```python
from build123d import *

# Parameters (mm, degrees)
SKIZZE1_R                       = 1.6
AUFSATZ_LINEAR_AUSTRAGEN1_DEPTH = 10


with BuildPart() as part:
    # Skizze1 → Aufsatz-Linear austragen1 (new body)
    with BuildSketch(Plane.XY):
        Polygon((5, 9.999223218), (4.999950827, 19.975708513), (-1, 19.999999998), (-1, 29.999223216), (5, 29.999223216), (4.999950827, 39.975708511), (-1, 39.999999996), (-1, 49.999223214), (5, 49.999223214), (4.999950827, 59.975708509), (-1, 59.999999994), (-1, 69.999223211), (5, 70), (4.999950827, 79.975708506), (-1, 79.999999991), (-1, 89.999223209), (5, 90), (4.999950827, 99.975708504), (-1, 99.999999989), (-1, 109.999223207), (5, 110), (4.999950827, 119.975708502), (-1, 119.999999987), (-1, 129.999223205), (5, 130), (4.999950827, 139.9757085), (-1, 139.999999985), (-1, 149.999223203), (5, 150), (4.999950827, 159.975708498), (-1, 159.999999983), (-1, 169.999223201), (5, 169.999223201), (4.999950827, 179.975708496), (-1, 179.999999981), (-1, 189.999223198), (5, 189.999223198), (4.999950827, 199.975708493), (-1, 199.999999978), (-1, 209.999223196), (5, 209.999223196), (4.999950827, 219.975708491), (5.0000043, 219.999971242), (35.0000043, 249.999971242), (45, 249.999971242), (45, 255.999971242), (55.0000043, 255.999971242), (55.0000043, 249.999971242), (65, 249.999971242), (65, 255.999971242), (75.0000043, 255.999971242), (75.0000043, 249.999971242), (85, 249.999971242), (85, 255.999971242), (95.0000043, 255.999971242), (95.0000043, 249.999971242), (105, 249.999971242), (105, 255.999971242), (115.0000043, 255.999971242), (115.0000043, 249.999971242), (125, 249.999971242), (125, 255.999971242), (135.0000043, 255.999971242), (135.0000043, 249.999971242), (145, 249.999971242), (145, 255.999971242), (155.0000043, 255.999971242), (155.0000043, 249.999971242), (165, 249.999971242), (165, 255.999971242), (175.0000043, 255.999971242), (175.0000043, 249.999971242), (185, 249.999971242), (185, 255.999971242), (195.0000043, 255.999971242), (195.0000043, 249.999971242), (205, 249.999971242), (205, 255.999971242), (215.0000043, 255.999971242), (215.0000043, 249.999971242), (225, 249.999971242), (225, 255.999971242), (235.0000043, 255.999971242), (235.0000043, 249.999971242), (245, 249.999971242), (245, 255.999971242), (255.0000043, 255.999971242), (255.0000043, 249.999971242), (265, 249.999971242), (265, 255.999971242), (275.0000043, 255.999971242), (275.0000043, 249.999971242), (305.0000043, 219.999969416), (304.999999999, 209.999969615), (311, 209.999967035), (311, 199.999972196), (305.0000043, 199.999972196), (304.999999999, 189.999972396), (311, 189.999969815), (311, 179.999974976), (305.0000043, 179.999974976), (304.999999999, 169.999975176), (311, 169.999972595), (311, 159.999977757), (305.0000043, 159.999977757), (304.999999999, 149.999977957), (311, 149.999975376), (311, 139.999980537), (305.0000043, 139.999980537), (304.999999999, 129.999980737), (311, 129.999978156), (311, 119.999983318), (305.0000043, 119.999983318), (304.999999999, 109.999983517), (311, 109.999980937), (311, 99.999986098), (305.0000043, 99.999986098), (304.999999999, 89.999986298), (311, 89.999983717), (311, 79.999988878), (305.0000043, 79.999988878), (304.999999999, 69.999989078), (311, 69.999986497), (311, 59.999991659), (305.0000043, 59.999991659), (304.999999999, 49.999991859), (311, 49.999989278), (311, 39.999994439), (305.0000043, 39.999994439), (304.999999999, 29.999994639), (311, 29.999992058), (311, 19.99999722), (305.0000043, 19.99999722), (304.999999999, 9.999997419), (311, 9.999994839), (311, 0), (305.0000043, 0), (4.956899878, 0), (-1, 0), (-1, 9.999223218), align=None)
        with Locations((290, 214.999999999)):
            Circle(SKIZZE1_R, mode=Mode.SUBTRACT)
        with Locations((280, 214.999999999)):
            Circle(SKIZZE1_R, mode=Mode.SUBTRACT)
        with Locations((20, 215)):
            Circle(SKIZZE1_R, mode=Mode.SUBTRACT)
        with Locations((30, 215)):
            Circle(SKIZZE1_R, mode=Mode.SUBTRACT)
        with Locations((20, 36)):
            Circle(SKIZZE1_R, mode=Mode.SUBTRACT)
        with Locations((155, 36)):
            Circle(SKIZZE1_R, mode=Mode.SUBTRACT)
        with Locations((290, 36)):
            Circle(SKIZZE1_R, mode=Mode.SUBTRACT)
        Polygon((275, 188.971165398), (245, 218.971165398), (65, 218.971165398), (35, 188.971165398), (35, 78.971165398), (275, 78.971165398), align=None, mode=Mode.SUBTRACT)
    extrude(amount=AUFSATZ_LINEAR_AUSTRAGEN1_DEPTH)


solid = part.part
```
Geometry check sheet. Reference: the model listing, model coordinates, mm. A direction names the side the tool comes from. Round coordinates to 2 decimals unless told otherwise and drop trailing zeros. Loops run counter-clockwise (first coordinate to the right, second up) from the corner with the lowest first, then second, coordinate; pieces in that order, holes last. Notation, with made-up numbers: (71.25, 36.25) - (87.25, 36.25) arc R33 cw to (87.25, 64.25) - close; hole circle Ø2 at (55.5, -19). An arc over 180 degrees is marked (long way). Write each question's results on one line, items separated by ' | '. Start each with the question number.
Q1. Cross-section at A-A on x = 118.5. Enter the section's corners in (y, z), and give its area (3 significant figures).
Q2. Cross-section at B-B on y = 203.5. Enter the section's corners in (x, z), and give its area (3 significant figures).
Q3. Cross-section at C-C on z = 2.5. State how many separate pieces and enclosed holes the cut face has, and give its area (3 significant figures).
Q4. Release check for a two-part mould opening along Y. For faces 1 (the flat face through (100, 250, 5)), 2 (the flat face through (305, 55, 5)), 3 (the flat face through (311, 85, 5)), 4 (the flat face through (156, 218.971, 5)) record: +Y half, -Y half, draft (parallel to the pull), parting line (faces both ways), or undercut.
Q5. Access from +Z, -Z, +X, -X, +Y, -Y to the whole of each face (thin tool, end or side, straight path). Record for faces 5 (the flat face through (305, 95, 5)), 6 (the flat face through (130, 256, 5)), 7 (the flat face through (305, 215, 5)), 8 (the flat face through (153, 78.971, 5)), 9 (the flat face through (200, 250, 5)).
Q6. Thickness scan on line 1 (Y direction, x = 20, z = 3); line 2 (Y direction, x = 162, z = 0.5); line 3 (X direction, y = 163, z = 4.5). Record the ranges inside material, lowest first. Write a range as [from, to].
Q7. Gauge pin test, flat ends, axial feed: P1, Ø5, axis at x = 1, z = 3.5, coming from the +Y side; P2, Ø3, axis at y = 114, z = 7, coming from the +X side; P3, Ø5, axis at x = 81.5, z = 5.5, coming from the +Y side. Record the tip position at first contact, or that the pin passes through.
Answers below:
1) outline: (0, 0) - (78.97, 0) - (78.97, 10) - (0, 10) - close; (218.97, 0) - (250, 0) - (250, 10) - (218.97, 10) - close | area: 1,100 mm²
2) outline: (-1, 0) - (49.53, 0) - (49.53, 10) - (-1, 10) - close; (260.47, 0) - (311, 0) - (311, 10) - (260.47, 10) - close | area: 1,010 mm²
3) separate pieces: 1 | enclosed holes: 8 | area: 43,400 mm²
4) face 1: +Y half | face 2: undercut | face 3: draft | face 4: undercut
5) face 5: +Z, -Z, +X | face 6: +Z, -Z, +X, -X, +Y | face 7: +Z, -Z, +X, +Y | face 8: +Z, -Z | face 9: +Z, -Z, +Y
6) line 1: y = [0, 34.4], [37.6, 213.4], [216.6, 235] | line 2: y = [0, 78.97], [218.97, 250] | line 3: x = [-1, 35], [275, 311]
7) P1: stops at y = 210 | P2: stops at x = 305 | P3: stops at y = 250
